Answer from the drawing. Dimensions are ordinates in mm from the lowest x, y and z of the part. A direction names the side the tool comes from. Coordinates: 2 decimals unless noted, no trailing zeros. Write each loop counter-clockwise with the first axis right and the second up, starting at its lowest first coordinate (ties: lowest second). Pieces come first, ordered by that corner, then holes.
1) Each of these flat-tipped pins is pushed along its axis until it touches: pin 1 Ø5 at (y, z) = (87, 4.5) entering from -X; pin 2 Ø10 at (y, z) = (140, 9.5) entering from -X; pin 3 Ø12 at (y, z) = (66, 8.5) entering from +X. Where does it stop, or does it pass through?
2) The part is cut by section A-A (z = 12.7). Determine the outline of the cut face in (x, y).
3) The part is cut by section D-D (x = 48.5). Determine the outline of the cut face in (y, z), then the cut area to 3 significant figures.
4) Which of the six approach directions +Z, -Z, +X, -X, +Y, -Y give full straight-line access (tool end or side, diameter ignored) to the marked faces 1 and 2?
5) The part is cut by section C-C (y = 32). Determine the outline of the cut face in (x, z).
6) Find the intervals of material crossed by line 1 (Y direction, x = 93.75, z = 12.7) (1 decimal); line 2 (Y direction, x = 93.25, z = 12.7) (1 decimal); line 3 (X direction, y = 111.5, z = 18.5), in increasing order.
7) The part is cut by section B-B (z = 5.5). Determine the outline of the cut face in (x, y).
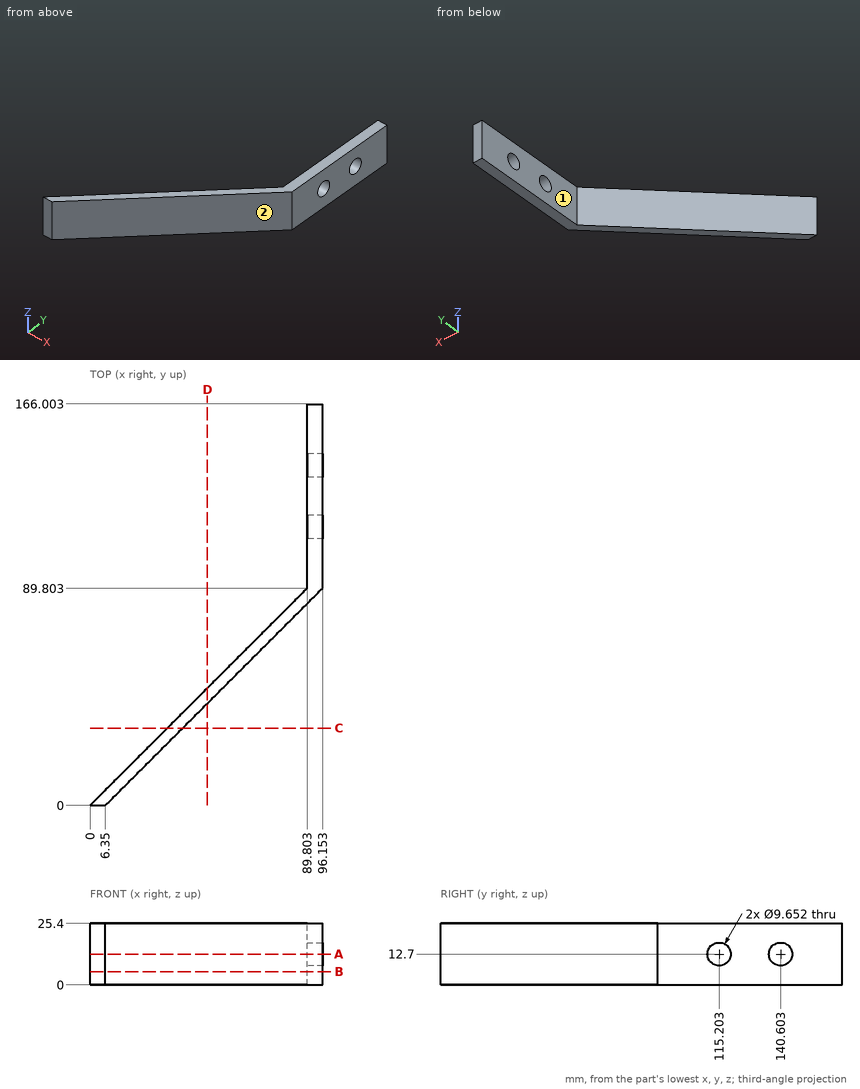
Reported:
1. pin 1: stops at x = 84.5
1. pin 2: stops at x = 89.8
1. pin 3: stops at x = 78.35
2. outline: (0, 0) - (6.35, 0) - (96.15, 89.8) - (96.15, 110.38) - (89.8, 110.38) - (89.8, 89.8) - close; (89.8, 120.03) - (96.15, 120.03) - (96.15, 135.78) - (89.8, 135.78) - close; (89.8, 145.43) - (96.15, 145.43) - (96.15, 166) - (89.8, 166) - close
3. outline: (42.15, 0) - (48.5, 0) - (48.5, 25.4) - (42.15, 25.4) - close
3. area: 161 mm2
4. face 1: +Z, -Z, -X, +Y
4. face 2: +Z, -Z, +X, -Y
5. outline: (32, 0) - (38.35, 0) - (38.35, 25.4) - (32, 25.4) - close
6. line 1: y = 87.4 to 110.4, 120 to 135.8, 145.4 to 166
6. line 2: y = 86.9 to 110.4, 120 to 135.8, 145.4 to 166
6. line 3: x = 89.8 to 96.15
7. outline: (0, 0) - (6.35, 0) - (96.15, 89.8) - (96.15, 166) - (89.8, 166) - (89.8, 89.8) - close
